The drawing under review shows one solid part. Ordinate dimensions are in mm from its lowest x, y, z. Round coordinates to 2 decimals unless told otherwise and drop trailing zeros. Write each loop counter-clockwise with the first axis right and the second up, starting at its lowest first coordinate (ties: lowest second). Pieces come first, ordered by that corner, then holes. Notation, with made-up numbers: (0.25, 30) -> (33.25, 30) arc R4 cw to (33.25, 36) -> close; hole circle Ø10 at (-38.75, 45). An arc over 180 degrees is marked (long way). Use CSV: the item, a comma, the result in double quotes. Start each with the question number.
1) Take a section at C-C, the plane z = 3.5. Give the boundary of the cut face in (x, y), then the cut area to 3 significant figures.
2) Wall thickness on probe 1 along X at (y, z) = (0.9, 15); probe 2 along Z at (x, y) = (132, 0.15); probe 3 along Z at (x, y) = (156, 0.6): over which ranges is each line inside the solid? List them lowest first. Write a range as [from, to].
3) For pin 1 Ø5 at (x, z) = (87.5, 24) entering from -Y; pin 2 Ø2.5 at (x, z) = (95, 25) entering from +Y, all flat-tipped, find the tip position at first contact; note any pin that passes through.
4) Take a section at A-A, the plane x = 139. Give the boundary of the cut face in (y, z).
5) Mouldability with a two-part tool opening along Y and no side actions: class the marked faces 1 and 2 as released by +Y, released by -Y, zero draft, split by the parting line, or undercut.
6) Take a section at B-B, the plane y = 0.5. State how many separate pieces and enclosed holes the cut face has, then the cut area to 3 significant figures.
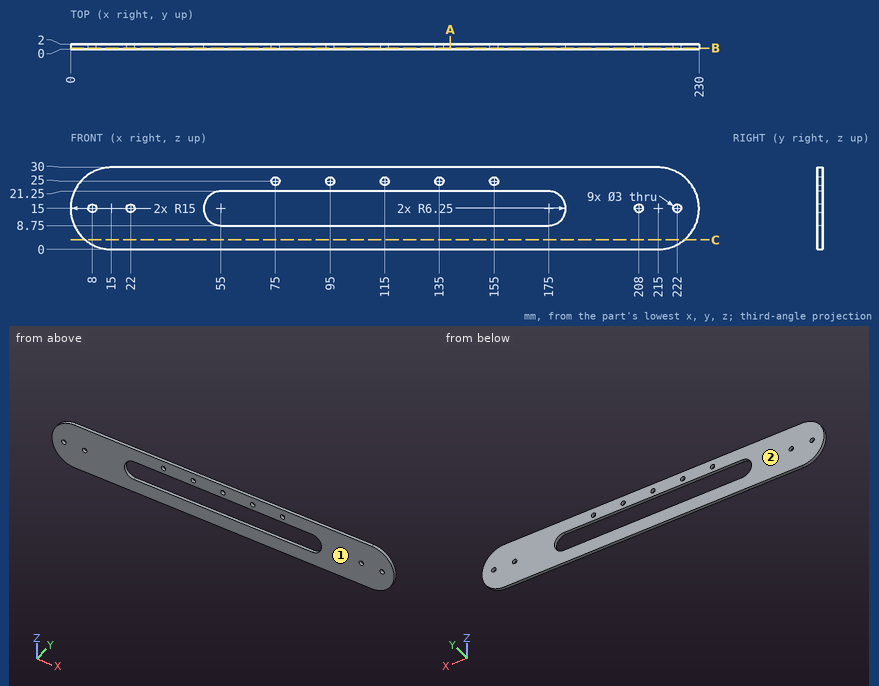
Values found:
1,outline,"(5.37, 0) -> (224.63, 0) -> (224.63, 2) -> (5.37, 2) -> close"
1,area,"439 mm²"
2,probe 1,"[0, 6.5], [9.5, 20.5], [23.5, 48.75], [181.25, 206.5], [209.5, 220.5], [223.5, 230]"
2,probe 2,"[0, 8.75], [21.25, 30]"
2,probe 3,"[0, 8.75], [21.25, 23.88], [26.12, 30]"
3,pin 1,"y = 0"
3,pin 2,"through"
4,outline,"(0, 0) -> (2, 0) -> (2, 8.75) -> (0, 8.75) -> close; (0, 21.25) -> (2, 21.25) -> (2, 30) -> (0, 30) -> close"
5,face 1,"released by -Y"
5,face 2,"released by +Y"
6,separate pieces,"1"
6,enclosed holes,"10"
6,area,"5,020 mm²"
